Source: CAD feature listing. Evaluate the final solid. Frame: model axes, mm. Face numbers are marked on the shaded views. A direction names the side the tool comes from. Give positions to 0.01 mm unless a question says otherwise; leave off trailing zeros. Loops run counter-clockwise (first coordinate to the right, second up) from the corner with the lowest first, then second, coordinate; pieces in that order, holes last.
```python
from build123d import *

# Parameters (mm, degrees)
SKETCH_1_R          = 11
EXTRUDE_1_DEPTH     = 23
SKETCH_2_R          = 20
EXTRUDE_2_DEPTH     = 5
SKETCH_3_R          = 8
CUT_EXTRUDE_1_DEPTH = 40.799497484
CHAMFER_1_SIZE      = 0.5
SKETCH_4_R          = 2.15
CUT_EXTRUDE_2_DEPTH = 40.799497484


with BuildPart() as part:
    # 草图1 → 凸台-拉伸1 (new body)
    with BuildSketch(Plane(origin=(0, 0, 0), x_dir=(1, 0, 0), z_dir=(0, 1, 0))):
        with Locations(Location((0, 0, 0), (0, 0, 270))):
            Circle(SKETCH_1_R)
    extrude(amount=EXTRUDE_1_DEPTH)

    # 草图2 → 凸台-拉伸2 (add)
    with BuildSketch(Plane(origin=(0, 23, 0), x_dir=(1, 0, 0), z_dir=(0, 1, 0))):
        with Locations(Location((0, 0, 0), (0, 0, 270))):
            Circle(SKETCH_2_R)
    extrude(amount=EXTRUDE_2_DEPTH)

    # 草图3 → 切除-拉伸1 (cut, through all)
    with BuildSketch(Plane(origin=(0, 28, 0), x_dir=(1, 0, 0), z_dir=(0, 1, 0))):
        with Locations(Location((0, 0, 0), (0, 0, 270))):
            Circle(SKETCH_3_R)
    extrude(amount=-CUT_EXTRUDE_1_DEPTH, mode=Mode.SUBTRACT)

    # 倒角1
    chamfer_1_edges = [part.edges().sort_by_distance(p)[0] for p in [
        (0, 0, -8),
        (0, 28, -8),
    ]]
    chamfer(chamfer_1_edges, length=CHAMFER_1_SIZE)

    # 草图4 → 切除-拉伸2 (cut, through all)
    with BuildSketch(Plane(origin=(0, 28, 0), x_dir=(1, 0, 0), z_dir=(0, 1, 0))):
        with Locations(Location((0, 15.5, 0), (0, 0, 270))):
            Circle(SKETCH_4_R)
        with Locations(Location((15.5, 0, 0), (0, 0, 270))):
            Circle(SKETCH_4_R)
        with Locations(Location((0, -15.5, 0), (0, 0, 270))):
            Circle(SKETCH_4_R)
        with Locations(Location((-15.5, 0, 0), (0, 0, 270))):
            Circle(SKETCH_4_R)
    extrude(amount=-CUT_EXTRUDE_2_DEPTH, mode=Mode.SUBTRACT)


solid = part.part
```
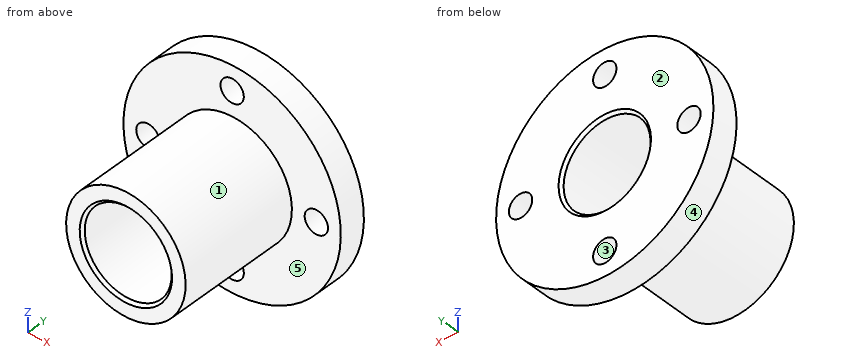
(1) Section B-B, the plane x = 0. Return the cut outline in (y, z), then the cut area to 4 significant figures.
A:
outline: (0, -11) - (23, -11) - (23, -13.35) - (28, -13.35) - (28, -8.5) - (27.5, -8) - (0.5, -8) - (0, -8.5) - close; (0, 8.5) - (0.5, 8) - (27.5, 8) - (28, 8.5) - (28, 13.35) - (23, 13.35) - (23, 11) - (0, 11) - close; (23, -20) - (28, -20) - (28, -17.65) - (23, -17.65) - close; (23, 17.65) - (28, 17.65) - (28, 20) - (23, 20) - close
area: 214.5 mm2
(2) Ray query, line 1 along X through (y, z) = (25.75, 0); line 2 along Y through (x, z) = (3.5, -11.5); line 3 along X through (y, z) = (25.1, 15.5). Return the intervals inside material, ascending.
A:
line 1: x = -20 to -17.65, -13.35 to -8, 8 to 13.35, 17.65 to 20
line 2: y = 23 to 28
line 3: x = -12.64 to -2.15, 2.15 to 12.64
(3) Section D-D, the plane z = -15.5. Return the cut outline in (x, y), then the cut area to 3 significant figures.
A:
outline: (-12.64, 23) - (-2.15, 23) - (-2.15, 28) - (-12.64, 28) - close; (2.15, 23) - (12.64, 23) - (12.64, 28) - (2.15, 28) - close
area: 105 mm2
(4) Reachability of the marked faces 4 and 5 from +Z, -Z, +X, -X, +Y, -Y: full face, straight path, thin tool, end or side. Return the list, or none.
A:
face 4: +Y, -Y
face 5: -Y
(5) Section C-C, the plane y = 25.5. Return the cut outline in (x, z), then the cut area to 3 significant figures.
A:
outline: circle Ø40 at (0, 0); hole circle Ø4.3 at (-15.5, 0); hole circle Ø16 at (0, 0); hole circle Ø4.3 at (0, -15.5); hole circle Ø4.3 at (0, 15.5); hole circle Ø4.3 at (15.5, 0)
area: 997 mm2
(6) Mould query, pull axis Z, two halves, no side actions, for the marked faces 1, 2 and 3. Classes: pulls with the +Z half, pulls with the -Z half, needs draft (parallel to the pull), parting line crosses it, or undercut.
A:
face 1: parting line crosses it
face 2: needs draft
face 3: undercut
(7) First-contact query: pin 1 (1 mm diameter, centred on x = -6.5, y = 23, fed in from +Z); pin 2 (2 mm diameter, centred on y = 5.5, z = 4, fed in from -X); pin 3 (2 mm diameter, centred on y = 10, z = -4.5, fed in from -X); pin 4 (7 mm diameter, centred on x = 15.5, z = 0, fed in from +Y). Flat tips, straight axial feed; report the tip coordinate or a pass-through.
A:
pin 1: stops at z = 19.08
pin 2: stops at x = -10.58
pin 3: stops at x = -10.43
pin 4: stops at y = 28
(8) Section A-A, the plane z = 0. Return the cut outline in (x, y), then the cut area to 4 significant figures.
A:
outline: (-20, 23) - (-17.65, 23) - (-17.65, 28) - (-20, 28) - close; (-13.35, 23) - (-11, 23) - (-11, 0) - (-8.5, 0) - (-8, 0.5) - (-8, 27.5) - (-8.5, 28) - (-13.35, 28) - close; (8, 0.5) - (8.5, 0) - (11, 0) - (11, 23) - (13.35, 23) - (13.35, 28) - (8.5, 28) - (8, 27.5) - close; (17.65, 23) - (20, 23) - (20, 28) - (17.65, 28) - close
area: 214.5 mm2
